from build123d import *

# Parameters (mm, degrees)
SKETCH1_W           = 426.72
SKETCH1_H           = 599.186
BOSS_EXTRUDE1_DEPTH = 167.64
FILLET1_R           = 60.8
SHELL4_T            = -6.35
BOSS_EXTRUDE3_START = -167.64
SKETCH7_W           = 450
SKETCH7_H           = 625
BOSS_EXTRUDE3_DEPTH = 20
CUT_EXTRUDE4_START  = 167.64
SKETCH8_R           = 91.297613413
CUT_EXTRUDE4_DEPTH  = 20
FILLET4_R           = 10


with BuildPart() as part:
    # Sketch1 → Boss-Extrude1 (new body)
    with BuildSketch(Plane(origin=(0, 0, 0), x_dir=(1, 0, 0), z_dir=(0, 1, 0))):
        Rectangle(SKETCH1_W, SKETCH1_H)
    extrude(amount=BOSS_EXTRUDE1_DEPTH)

    # Fillet1
    fillet1_edges = [part.edges().sort_by_distance(p)[0] for p in [
        (0, 0, 299.593),
        (-213.36, 0, 0),
        (0, 0, -299.593),
        (213.36, 0, 0),
    ]]
    fillet(fillet1_edges, radius=FILLET1_R)

    # Shell4
    shell4_openings = [part.faces().sort_by_distance(p)[0] for p in [
        (0, 167.64, 0),
    ]]
    offset(amount=SHELL4_T, openings=shell4_openings)

    # Sketch7 → Boss-Extrude3 (add)
    with BuildSketch(Plane.XZ.offset(BOSS_EXTRUDE3_START)):
        Rectangle(SKETCH7_W, SKETCH7_H)
    extrude(amount=-BOSS_EXTRUDE3_DEPTH)

    # Sketch8 → Cut-Extrude4 (cut)
    with BuildSketch(Plane(origin=(0, 0, 0), x_dir=(1, 0, 0), z_dir=(0, 1, 0)).offset(CUT_EXTRUDE4_START)):
        with Locations(Location((0, -156.25, 0), (0, 0, 90))):
            Circle(SKETCH8_R)
        with Locations(Location((0, 156.25, 0), (0, 0, 90))):
            Circle(SKETCH8_R)
    extrude(amount=CUT_EXTRUDE4_DEPTH, mode=Mode.SUBTRACT)

    # Fillet4
    fillet4_edges = [part.edges().sort_by_distance(p)[0] for p in [
        (-225, 187.64, 0),
        (-225, 177.64, -312.5),
        (0, 187.64, 312.5),
        (-225, 177.64, 312.5),
        (225, 187.64, 0),
        (225, 177.64, 312.5),
        (0, 187.64, -312.5),
        (225, 177.64, -312.5),
    ]]
    fillet(fillet4_edges, radius=FILLET4_R)


solid = part.part
Work out the finished part from the listing and answer in its coordinate system (mm). A direction names the side the tool comes from. Give positions to 0.01 mm unless a question says otherwise; leave off trailing zeros. Loops run counter-clockwise (first coordinate to the right, second up) from the corner with the lowest first, then second, coordinate; pieces in that order, holes last. Notation, with made-up numbers: (-22.5, -3.75) -> (18.5, -3.75) arc R19 cw to (18.5, 2.25) -> close; hole circle Ø2 at (-7, -22). An arc over 180 degrees is marked (long way). Use a Markdown table: item, result. Add a question column.
1) The part is cut by section A-A, the plane x = 0. Determine the outline of the cut face in (y, z), plus the area to 3 significant figures.
2) Consider line 1 along Y through (x, z) = (92, -219.5); line 2 along X through (y, z) = (93, -42); line 3 along X through (y, z) = (174, 156). Determine where each line is inside the solid, lowest interval first.
3) The part is cut by section D-D, the plane z = -271. Determine the outline of the cut face in (x, y).
4) Each of these flat-tipped pins is pushed along its axis until it touches: P1, Ø10, axis at y = 48.5, z = 216, coming from the +X side; P2, Ø12, axis at y = 142.5, z = -0.5, coming from the +X side; P3, Ø6, axis at x = 125.5, y = 71.5, coming from the +Z side; P4, Ø10, axis at x = -75.5, z = 240, coming from the -Y side. Where does it stop, or does it pass through?
5) The part is cut by section C-C, the plane z = 156.25. Determine the outline of the cut face in (x, y), plus the area to 3 significant figures.
6) Which of the six approach directions +Z, -Z, +X, -X, +Y, -Y give full straight-line access (tool end or side, diameter ignored) to faces 1 (the cylindrical face through (-4.01, 177.5, 247.46)), 2 (the flat face through (207.01, 113, 4)), 3 (the flat face through (-213.36, 113, 4))?
7) For a pull along X with two mould halves and no side action, classify faces 4 (the cylindrical face through (2.898, 22.724, 277.716)), 5 (the cylindrical face through (-196.02, 18.28, -4.19)), 6 (the cylindrical face through (2.987, 18.283, -282.255)) as +X half, -X half, draft (parallel to the pull), parting line (faces both ways), or undercut.
8) The part is cut by section B-B, the plane y = 145. Determine the outline of the cut face in (x, z), plus the area to 3 significant figures.
Reported:
| question | item | result |
|---|---|---|
| 1 | outline | (0, -238.79) arc R60.8 ccw to (60.8, -299.59) -> (167.64, -299.59) -> (167.64, -312.5) -> (177.64, -312.5) arc R10 ccw to (187.64, -302.5) -> (187.64, -247.55) -> (167.64, -247.55) -> (167.64, -293.24) -> (60.8, -293.24) arc R54.45 cw to (6.35, -238.79) -> (6.35, 238.79) arc R54.45 cw to (60.8, 293.24) -> (167.64, 293.24) -> (167.64, 247.55) -> (187.64, 247.55) -> (187.64, 302.5) arc R10 ccw to (177.64, 312.5) -> (167.64, 312.5) -> (167.64, 299.59) -> (60.8, 299.59) arc R60.8 ccw to (0, 238.79) -> close; (167.64, -64.95) -> (187.64, -64.95) -> (187.64, 64.95) -> (167.64, 64.95) -> close |
| 1 | area | 10,700 mm^2 |
| 2 | line 1 | y = 0 to 6.35, 167.64 to 187.64 |
| 2 | line 2 | x = -213.36 to -207.01, 207.01 to 213.36 |
| 2 | line 3 | x = -225 to -91.3, 91.3 to 225 |
| 3 | outline | (-225, 167.64) -> (-213.36, 167.64) -> (-213.36, 60.8) arc R60.8 ccw to (-184.77, 9.23) -> (184.77, 9.23) arc R60.8 ccw to (213.36, 60.8) -> (213.36, 167.64) -> (225, 167.64) -> (225, 177.64) arc R10 ccw to (215, 187.64) -> (-215, 187.64) arc R10 ccw to (-225, 177.64) -> close; hole (-207.01, 60.8) arc R54.45 ccw to (-184.77, 16.9) -> (184.77, 16.9) arc R54.45 ccw to (207.01, 60.8) -> (207.01, 167.64) -> (-207.01, 167.64) -> close |
| 4 | P1 | stops at x = 212.92 |
| 4 | P2 | stops at x = 213.36 |
| 4 | P3 | stops at z = 299.59 |
| 4 | P4 | stops at y = 0 |
| 5 | outline | (-225, 167.64) -> (-213.36, 167.64) -> (-213.36, 60.8) arc R60.8 ccw to (-152.56, 0) -> (152.56, 0) arc R60.8 ccw to (213.36, 60.8) -> (213.36, 167.64) -> (225, 167.64) -> (225, 177.64) arc R10 ccw to (215, 187.64) -> (91.3, 187.64) -> (91.3, 167.64) -> (207.01, 167.64) -> (207.01, 60.8) arc R54.45 cw to (152.56, 6.35) -> (-152.56, 6.35) arc R54.45 cw to (-207.01, 60.8) -> (-207.01, 167.64) -> (-91.3, 167.64) -> (-91.3, 187.64) -> (-215, 187.64) arc R10 ccw to (-225, 177.64) -> close |
| 5 | area | 9,750 mm^2 |
| 6 | face 1 | +Y |
| 6 | face 2 | none |
| 6 | face 3 | +Z, -Z, -X, -Y |
| 7 | face 4 | undercut |
| 7 | face 5 | -X half |
| 7 | face 6 | draft |
| 8 | outline | (-213.36, -299.59) -> (213.36, -299.59) -> (213.36, 299.59) -> (-213.36, 299.59) -> close; hole (-207.01, -293.24) -> (207.01, -293.24) -> (207.01, 293.24) -> (-207.01, 293.24) -> close |
| 8 | area | 12,900 mm^2 |
